Can you work these out from the model? Positions are in its coordinate system, mm. Face numbers are marked on the shaded views. A direction names the side the tool comes from. Coordinates: 2 decimals unless noted, no trailing zeros. Loops run counter-clockwise (first coordinate to the right, second up) from the corner with the lowest first, then second, coordinate; pieces in that order, holes last.
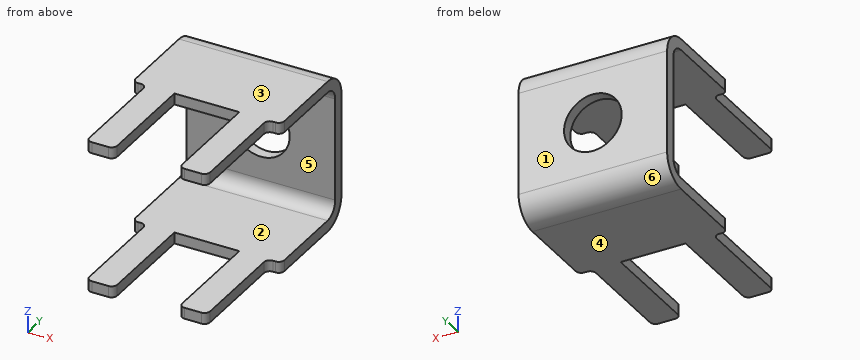
```python
from build123d import *

# Parameters (mm, degrees)
SKETCH_1_W                         = 8
SKETCH_1_H                         = 8.2
SM_BASE_FLANGE_1_DEPTH             = 0.6
SM_EDGE_FLANGE_1_STRIP_W           = 3.8732
SM_EDGE_FLANGE_1_STRIP_H           = 0.6
SM_EDGE_FLANGE_1_STRIP_CUT_DEPTH   = 8
SM_EDGE_FLANGE_1_STRIP_2_W         = 3.8732
SM_EDGE_FLANGE_1_STRIP_2_H         = 0.6
SM_EDGE_FLANGE_1_STRIP_CUT_2_DEPTH = 8
SM_EDGE_FLANGE_1_DEPTH             = 8
SM_EDGE_FLANGE_1_BEND_DEPTH        = 8
SKETCH_10_OUTSIDE_W                = 13.26
SKETCH_10_OUTSIDE_H                = 13.46
SKETCH_10_OUTSIDE_W_2              = 1.5
SKETCH_10_OUTSIDE_H_2              = 9.508037294
CUT_EXTRUDE_1_DEPTH                = 5.8
FILLET_1_R                         = 0.3
FILLET_2_R                         = 0.3
SKETCH_11_R                        = 1.55
CUT_EXTRUDE_2_DEPTH                = 5.8


# Sheet-metal steps are written as plain solids
with BuildPart() as part:
    # Sketch 1 → 基体-法兰1 (new body)
    with BuildSketch(Plane(origin=(0, 0, 0), x_dir=(1, 0, 0), z_dir=(0, 1, 0))):
        Rectangle(SKETCH_1_W, SKETCH_1_H)
    extrude(amount=-SM_BASE_FLANGE_1_DEPTH)

    # 边线-法兰1 strip (across the edge) → 边线-法兰1 strip cut (cut)
    with BuildSketch(Plane(origin=(4, -0.6, 4.1), x_dir=(0, 0, -1), z_dir=(-1, 0, 0))):
        with Locations((-0.6, -0.3)):
            Rectangle(SM_EDGE_FLANGE_1_STRIP_W, SM_EDGE_FLANGE_1_STRIP_H)
    extrude(amount=SM_EDGE_FLANGE_1_STRIP_CUT_DEPTH, mode=Mode.SUBTRACT)

    # 边线-法兰1 strip 2 (across the edge) → 边线-法兰1 strip cut 2 (cut)
    with BuildSketch(Plane(origin=(-4, -0.6, -4.1), x_dir=(0, 0, 1), z_dir=(1, 0, 0))):
        with Locations((-0.6, -0.3)):
            Rectangle(SM_EDGE_FLANGE_1_STRIP_2_W, SM_EDGE_FLANGE_1_STRIP_2_H)
    extrude(amount=SM_EDGE_FLANGE_1_STRIP_CUT_2_DEPTH, mode=Mode.SUBTRACT)

    # 边线-法兰1 section (across the edge) → 边线-法兰1 (add)
    with BuildSketch(Plane(origin=(4, -0.6, 4.1), x_dir=(0, 0, -1), z_dir=(-1, 0, 0))):
        with BuildLine():
            Line((0, 0.7366), (0, 11))
            Line((0, 11), (0.6, 11))
            Line((0.6, 11), (0.6, 0.7366))
            ThreePointArc((0.6, 0.7366), (0.815745145, 0.215745145), (1.3366, 0))
            Line((1.3366, 0), (1.3366, -0.6))
            ThreePointArc((1.3366, -0.6), (0.391481076, -0.208518924), (0, 0.7366))
        make_face()
    extrude(amount=SM_EDGE_FLANGE_1_DEPTH)

    # 边线-法兰1 section 2 (across the edge) → 边线-法兰1 bend (add)
    with BuildSketch(Plane(origin=(-4, -0.6, -4.1), x_dir=(0, 0, 1), z_dir=(1, 0, 0))):
        with BuildLine():
            Line((0, 0.7366), (0, 11))
            Line((0, 11), (0.6, 11))
            Line((0.6, 11), (0.6, 0.7366))
            ThreePointArc((0.6, 0.7366), (0.815745145, 0.215745145), (1.3366, 0))
            Line((1.3366, 0), (1.3366, -0.6))
            ThreePointArc((1.3366, -0.6), (0.391481076, -0.208518924), (0, 0.7366))
        make_face()
    extrude(amount=SM_EDGE_FLANGE_1_BEND_DEPTH)

    # 草图10 outside → 切除-拉伸1 (cut)
    with BuildSketch(Plane.XZ.offset(11.6)):
        Rectangle(SKETCH_10_OUTSIDE_W, SKETCH_10_OUTSIDE_H)
        with Locations((-2.5, -0.421070223)):
            Rectangle(SKETCH_10_OUTSIDE_W_2, SKETCH_10_OUTSIDE_H_2, mode=Mode.SUBTRACT)
        with Locations((2.5, -0.421070223)):
            Rectangle(SKETCH_10_OUTSIDE_W_2, SKETCH_10_OUTSIDE_H_2, mode=Mode.SUBTRACT)
    extrude(amount=-CUT_EXTRUDE_1_DEPTH, mode=Mode.SUBTRACT)

    # 圆角1
    fillet_1_edges = [part.edges().sort_by_distance(p)[0] for p in [
        (-3.25, -11.6, 3.8),
        (-1.75, -11.6, 3.8),
        (3.25, -11.6, 3.8),
        (1.75, -11.6, 3.8),
        (1.75, -11.6, -3.8),
        (3.25, -11.6, -3.8),
        (-1.75, -11.6, -3.8),
        (-3.25, -11.6, -3.8),
    ]]
    fillet(fillet_1_edges, radius=FILLET_1_R)

    # 圆角2
    fillet_2_edges = [part.edges().sort_by_distance(p)[0] for p in [
        (3.25, -5.8, 3.8),
        (-3.25, -5.8, 3.8),
        (-3.25, -5.8, -3.8),
        (3.25, -5.8, -3.8),
        (-4, -5.8, 3.8),
        (-4, -5.8, -3.8),
        (4, -5.8, -3.8),
        (4, -5.8, 3.8),
    ]]
    fillet(fillet_2_edges, radius=FILLET_2_R)

    # 草图11 → 切除-拉伸2 (cut)
    with BuildSketch(Plane(origin=(0, 0, 0), x_dir=(1, 0, 0), z_dir=(0, 1, 0))):
        with Locations(Location((0, 0, 0), (0, 0, 270))):
            Circle(SKETCH_11_R)
    extrude(amount=-CUT_EXTRUDE_2_DEPTH, mode=Mode.SUBTRACT)


solid = part.part
```
(1) I want a section at D-D on y = -5. Write out the boundary of the cut face in (x, z), then the cut area to 3 significant figures.
Check values:
outline: (-4, -4.1) - (4, -4.1) - (4, -3.5) - (-4, -3.5) - close; (-4, 3.5) - (4, 3.5) - (4, 4.1) - (-4, 4.1) - close
area: 9.60 mm2
(2) I want a section at A-A on z = 0. Write out the boundary of the cut face in (x, y), then the cut area to 3 significant figures.
Check values:
outline: (-4, -0.6) - (-1.55, -0.6) - (-1.55, 0) - (-4, 0) - close; (1.55, -0.6) - (4, -0.6) - (4, 0) - (1.55, 0) - close
area: 2.94 mm2
(3) I'm going to push flat-ended pins straight in: pin 1 (0.7 mm diameter, centred on y = -8, z = -4, fed in from +X); pin 2 (0.7 mm diameter, centred on y = -7.5, z = -3.5, fed in from -X); pin 3 (2.5 mm diameter, centred on x = 0, z = 0, fed in from -Y); pin 4 (4 mm diameter, centred on x = 3, z = -0.5, fed in from -Y). Where does each tip first touch, or does it pass through?
Check values:
pin 1: stops at x = 3.25
pin 2: stops at x = -3.25
pin 3: passes through
pin 4: stops at y = -0.6
(4) I want a section at B-B on x = 0. Write out the boundary of the cut face in (y, z), then the cut area to 3 significant figures.
Check values:
outline: (-5.8, -4.1) - (-1.34, -4.1) arc R1.34 ccw to (0, -2.76) - (0, -1.55) - (-0.6, -1.55) - (-0.6, -2.76) arc R0.74 cw to (-1.34, -3.5) - (-5.8, -3.5) - close; (-5.8, 3.5) - (-1.34, 3.5) arc R0.74 cw to (-0.6, 2.76) - (-0.6, 1.55) - (0, 1.55) - (0, 2.76) arc R1.34 ccw to (-1.34, 4.1) - (-5.8, 4.1) - close
area: 8.77 mm2
(5) If I drill on probe 1 along X at (y, z) = (-0.4, 0); probe 2 along Z at (x, y) = (3.5, -1.5); probe 3 along Y at (x, z) = (1.75, -1.5), over which ranges is the centre line in solid material (lowest first)?
Check values:
probe 1: x = -4 to -1.55, 1.55 to 4
probe 2: z = -4.1 to -3.5, 3.5 to 4.1
probe 3: y = -0.6 to 0
(6) I want a section at C-C on y = -8. Write out the boundary of the cut face in (x, z).
Check values:
outline: (-3.25, -4.1) - (-1.75, -4.1) - (-1.75, -3.5) - (-3.25, -3.5) - close; (-3.25, 3.5) - (-1.75, 3.5) - (-1.75, 4.1) - (-3.25, 4.1) - close; (1.75, -4.1) - (3.25, -4.1) - (3.25, -3.5) - (1.75, -3.5) - close; (1.75, 3.5) - (3.25, 3.5) - (3.25, 4.1) - (1.75, 4.1) - close
(7) Which directions (+Z, -Z, +X, -X, +Y, -Y) give clear straight access to the entire face, cutting with the end or side of a thin tool? Please do the marked faces 5 and 6.
Check values:
face 5: +X, -X, -Y
face 6: -Z, +X, -X, +Y
(8) If we mould it in two halves opening along Z, with no side actions, what happens to the marked faces 1, 2, 3 and 4? For each: released by +Z, released by -Z, zero draft, split by the parting line, or undercut.
Check values:
face 1: zero draft
face 2: undercut
face 3: released by +Z
face 4: released by -Z
